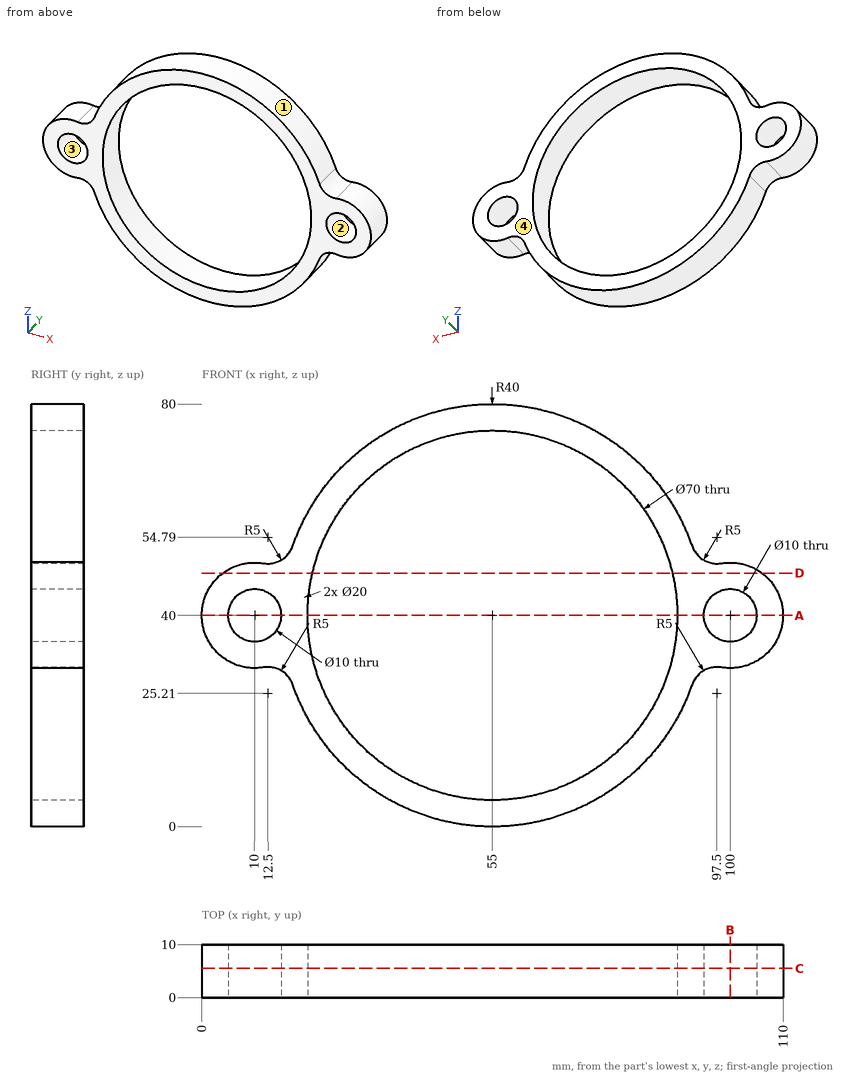
Part print with two shaded views. Sizes in mm from the minimum x, y, z corner. Coordinates: 2 decimals unless noted, no trailing zeros. Write each loop counter-clockwise with the first axis right and the second up, starting at its lowest first coordinate (ties: lowest second). Pieces come first, ordered by that corner, then holes. Notation, with made-up numbers: (51.25, -34.5) - (67.25, -34.5) arc R14 ccw to (67.25, -19.5) - close; hole circle Ø8 at (40, 4). An arc over 180 degrees is marked (long way). Use a Markdown table: item, result. Add a question column.
Item 1: Band-saw the part on A-A, the plane z = 40. Write the cut outline in (x, y).
Item 2: Drop flat-ended pins along their axis: pin 1 (3 mm diameter, centred on x = 22, y = 7.5, fed in from +Z); pin 2 (5 mm diameter, centred on y = 6.5, z = 12, fed in from +X); pin 3 (2 mm diameter, centred on x = 32.5, y = 6, fed in from -Z). Give the stop position or say it passes through.
Item 3: Band-saw the part on B-B, the plane x = 100. Write the cut outline in (y, z).
Item 4: Drill centre lines: line 1 along Z through (x, y) = (31.5, 8.75); line 2 along X through (y, z) = (7, 61) (1 decimal); line 3 along Z through (x, y) = (75.5, 9.75). Where is each one in solid material? Low to high.
Item 5: Two-plate mould, pull along X, no slides. Class the marked faces 1, 2, 3 and 4: pulls with the +X half, pulls with the -X half, needs draft (parallel to the pull), parting line crosses it, or undercut.
Item 6: Band-saw the part on C-C, the plane y = 5.5. Write the cut outline in (x, z), and give its area (3 significant figures).
Item 7: Band-saw the part on D-D, the plane z = 48. Write the cut outline in (x, y).
A:
| question | item | result |
|---|---|---|
| 1 | outline | (0, 0) - (5, 0) - (5, 10) - (0, 10) - close; (15, 0) - (20, 0) - (20, 10) - (15, 10) - close; (90, 0) - (95, 0) - (95, 10) - (90, 10) - close; (105, 0) - (110, 0) - (110, 10) - (105, 10) - close |
| 2 | pin 1 | stops at z = 64.65 |
| 2 | pin 2 | stops at x = 85.82 |
| 2 | pin 3 | stops at z = 6.27 |
| 3 | outline | (0, 30) - (10, 30) - (10, 35) - (0, 35) - close; (0, 45) - (10, 45) - (10, 50) - (0, 50) - close |
| 4 | line 1 | z = 7.63 to 14.06, 65.94 to 72.37 |
| 4 | line 2 | x = 21 to 27, 83 to 89 |
| 4 | line 3 | z = 5.65 to 11.63, 68.37 to 74.35 |
| 5 | face 1 | parting line crosses it |
| 5 | face 2 | undercut |
| 5 | face 3 | undercut |
| 5 | face 4 | needs draft |
| 6 | outline | (11.67, 30.14) arc R5 cw to (17.22, 26.85) arc R40 ccw to (92.78, 26.85) arc R5 cw to (98.33, 30.14) arc R10 ccw (long way) to (98.33, 49.86) arc R5 cw to (92.78, 53.15) arc R40 ccw to (17.22, 53.15) arc R5 cw to (11.67, 49.86) arc R10 ccw (long way) to start; hole circle Ø10 at (10, 40); hole circle Ø70 at (55, 40); hole circle Ø10 at (100, 40) |
| 6 | area | 1,560 mm² |
| 7 | outline | (4, 0) - (20.93, 0) - (20.93, 10) - (4, 10) - close; (89.07, 0) - (106, 0) - (106, 10) - (89.07, 10) - close |
